Here's how the part is built. I have some questions about the finished solid (model axes, mm). A direction names the side the tool comes from. Coordinates: 2 decimals unless noted, no trailing zeros. Write each loop counter-clockwise with the first axis right and the second up, starting at its lowest first coordinate (ties: lowest second). Pieces come first, ordered by that corner, then holes. Notation, with made-up numbers: M 61.5,23 L 112.5,23 A15 cw 112.5,46 Z; hole C 51.5,24 d4. An arc over 180 degrees is marked long. Write each question's results on one line, items separated by ' | '. Start each with the question number.
Autodesk Inventor part; units mm, degrees
ref_plane "YZ Plane" through (0, 0, 0) normal (1, 0, 0) x (0, 1, 0)
ref_plane "XZ Plane" through (0, 0, 0) normal (0, 1, 0) x (-1, 0, 0)
ref_plane "XY Plane" through (0, 0, 0) normal (0, 0, 1) x (1, 0, 0)
sketch "Skizze1" plane through (0, 0, 0) normal (1, 0, 0) x (0, 1, 0)
  line L0 (-25.5, -32.5) -> (25.5, -32.5)
  line L1 (25.5, -32.5) -> (25.5, 32.5)
  line L2 (25.5, 32.5) -> (-25.5, 32.5)
  line L3 (-25.5, 32.5) -> (-25.5, -32.5)
  line L4 (-25.5, -32.5) -> (25.5, 32.5) construction
  line L5 (25.5, -32.5) -> (-25.5, 32.5) construction
  point P0 (0, 0)
  dimension "d0" = 51
  dimension "d1" = 65
extrude "Extrusion1" add sketch "Skizze1" along normal blind 9
fillet "Rundung1" radius 3 4 edges at (9, 25.5, 0) (0, 25.5, 0) (9, -25.5, 0) (0, -25.5, 0)
fillet "Rundung2" radius 1 16 edges at (8.1213, -24.6213, 32.5) (4.5, -25.5, 32.5) (0.8787, -24.6213, 32.5) (0, 0, 32.5) (0.8787, 24.6213, 32.5) (4.5, 25.5, 32.5) (8.1213, 24.6213, 32.5) (9, 0, 32.5) (8.1213, 24.6213, -32.5) (4.5, 25.5, -32.5) (0.8787, 24.6213, -32.5) (0, 0, -32.5) (0.8787, -24.6213, -32.5) (4.5, -25.5, -32.5) (8.1213, -24.6213, -32.5) (9, 0, -32.5)
sketch "Skizze2" plane through (0, 0, 0) normal (-1, 0, 0) x (0, 0, 1)
  circle A0 centre (0, 0) radius 5
  dimension "d6" = 10
extrude "Extrusion2" add sketch "Skizze2" along normal blind 0.5
properties part number "PKCell 3.7V 2500mAh"
1) I want a section at D-D, the plane y = 0. Write out the boundary of the cut face in (x, z), then the cut area to 3 significant figures.
2) For faces 1 (the cylindrical face through (-0.25, 4.88, -1.08)), 2 (the flat face through (4, 25.5, 0)), which set-ups out of +Z, -Z, +X, -X, +Y, -Y let a thin tool reach every point of the face, with its end or its side?
3) I want a section at C-C, the plane z = 11. Write out the boundary of the cut face in (x, y).
4) I want a section at B-B, the plane y = -21.5. Write out the boundary of the cut face in (x, z).
5) Please list where these lines run through material, in increasing order: line 1 (X direction, y = 14, z = -5); line 2 (Z direction, x = 8.25, y = -0.5); line 3 (Y direction, x = 1.5, z = -26). Write a range as [from, to].
6) I want a section at A-A, the plane z = 0. Write out the boundary of the cut face in (x, y).
7) For pin 1 Ø13.5 at (y, z) = (-4, -11.5) entering from -X; pin 2 Ø1 at (x, z) = (2, 2.5) entering from -Y, each with a flat end and sliding along its axis, tell me the tip position at first contact or that it passes through.
Output:
1) outline: M -0.5,-5 L 0,-5 L 0,-31.5 A1 ccw 1,-32.5 L 8,-32.5 A1 ccw 9,-31.5 L 9,31.5 A1 ccw 8,32.5 L 1,32.5 A1 ccw 0,31.5 L 0,5 L -0.5,5 Z | area: 589 mm2
2) face 1: -X | face 2: +Z, -Z, +X, -X, +Y
3) outline: M 0,-22.5 A3 ccw 3,-25.5 L 6,-25.5 A3 ccw 9,-22.5 L 9,22.5 A3 ccw 6,25.5 L 3,25.5 A3 ccw 0,22.5 Z
4) outline: M 0,-31.5 A1 ccw 1,-32.5 L 8,-32.5 A1 ccw 9,-31.5 L 9,31.5 A1 ccw 8,32.5 L 1,32.5 A1 ccw 0,31.5 Z
5) line 1: x = [0, 9] | line 2: z = [-32.47, 32.47] | line 3: y = [-25.1, 25.1]
6) outline: M -0.5,-5 L 0,-5 L 0,-22.5 A3 ccw 3,-25.5 L 6,-25.5 A3 ccw 9,-22.5 L 9,22.5 A3 ccw 6,25.5 L 3,25.5 A3 ccw 0,22.5 L 0,5 L -0.5,5 Z
7) pin 1: stops at x = 0 | pin 2: stops at y = -25.46
